Input: part model. Units: mm. Frame: model coordinates. A direction names the side the tool comes from. Round coordinates to 2 decimals unless told otherwise and drop trailing zeros. Loops run counter-clockwise (first coordinate to the right, second up) from the corner with the lowest first, then second, coordinate; pieces in that order, holes last. Notation, with made-up numbers: M -13,29 L 33,29 A15 cw 33,57 Z; hole C 59,-9.5 d3. An arc over 180 degrees is marked long. Return JSON: item names as keys, results as strings. Group by question number.
1) Section D-D (y = -54). Output: boundary loops of the cut face in (x, z).
2) Section B-B (x = 0). Count the separate pieces of the cut face and the enclosed holes in it, plus the area to 3 significant figures.
3) Contact query for flat-ended pins moving along their axis: P1, Ø3, axis at x = 0, z = 0, coming from the +Y side; P2, Ø4, axis at y = -53.5, z = 1.5, coming from the -X side; P3, Ø2, axis at x = 0, y = -56, coming from the +Z side; P4, Ø1.5, axis at x = -3.5, z = 3, coming from the +Y side. Output: stop coordinate, or through.
4) Mould query, pull axis X, two halves, no side actions, for faces 4 (the face through (5.94, -73.819, -1.38)), 5 (the face through (1.38, -75.1, -6.2)), 6 (the face through (-0.05, -41.78, 4.91)). Classes: +X half, -X half, draft (parallel to the pull), parting line (faces both ways), or undercut.
5) Access query for faces 1 (the face through (-5.669, -74.307, 1.785)), 2 (the face through (-0.05, -41.78, -4.8)), 3 (the face through (0, -59, 6.35)). Directions: +Z, -Z, +X, -X, +Y, -Y. A direction counts if a zero-diameter tool reaches every point of the face in a straight line with its end or side. Return the directions, or none.
6) Section A-A (y = -41). Output: boundary loops of the cut face in (x, z).
7) Section C-C (y = -13). Output: boundary loops of the cut face in (x, z).
8) Material intervals for line 1 (X direction, y = -17.75, z = 0); line 2 (X direction, y = -6.5, z = 0); line 3 (Y direction, x = 0.75, z = -6.25), sorted ascending. Write a range as from..to.
from build123d import *

# Parameters (mm, degrees)
F0_R     = 6.35
F0_R_2   = 2.4892
F1_DEPTH = 17.4625
F2_R     = 2.4892
F3_DEPTH = 27.78125
F5_DEPTH = 15.876
F7_DEPTH = 30.1625


with BuildPart() as f1:
    # F0 (on Front) → F1 (new body)
    with BuildSketch(Plane.XZ):
        Circle(F0_R)
        Circle(F0_R_2, mode=Mode.SUBTRACT)
    extrude(amount=F1_DEPTH)

    # F2 (on face) → F3 (join)
    with BuildSketch(Plane.XZ.offset(17.4625)):
        Polygon((4.5827177617, 7.9375), (-4.5827177617, 7.9375), (-9.1654355234, 0), (-4.5827177617, -7.9375), (4.5827177617, -7.9375), (9.1654355234, 0), align=None)
        Circle(F2_R, mode=Mode.SUBTRACT)
    extrude(amount=F3_DEPTH)

    # F4 (on face) → F5 (cut, through all)
    with BuildSketch(Plane.XY.offset(7.9375)):
        with BuildLine():
            ThreePointArc((2.4892, -23.415625), (0, -20.926425), (-2.4892, -23.415625))
            Line((-2.4892, -23.415625), (-2.4892, -39.290625))
            ThreePointArc((-2.4892, -39.290625), (0, -41.779825), (2.4892, -39.290625))
            Line((2.4892, -39.290625), (2.4892, -23.415625))
        make_face()
    extrude(amount=-F5_DEPTH, mode=Mode.SUBTRACT)

    # F6 (on face) → F7 (join)
    with BuildSketch(Plane.XZ.offset(45.24375)):
        Polygon((-3.6661742094, -6.35), (3.6661742094, -6.35), (7.3323484187, 0), (3.6661742094, 6.35), (-3.6661742094, 6.35), (-7.3323484187, 0), align=None)
    extrude(amount=F7_DEPTH)

    # F8 (on Top) → F9 (revolve, cut)
    with BuildSketch(Plane.XY):
        Polygon((-7.3323484187, -75.40625), (-6.35, -75.40625), (-6.35, -74.80935), (-5.9436, -74.80935), (-5.9436, -73.81875), (-7.3323484187, -73.81875), align=None)
        Polygon((6.35, -74.80935), (6.35, -75.40625), (7.3323484187, -75.40625), (7.3323484187, -73.81875), (5.9436, -73.81875), (5.9436, -74.80935), align=None)
        Polygon((7.3323484187, -1.5875), (7.3323484187, 0), (6.35, 0), (6.35, -0.5969), (5.9436, -0.5969), (5.9436, -1.5875), align=None)
        Polygon((-5.9436, -0.5969), (-6.35, -0.5969), (-6.35, 0), (-7.3323484187, 0), (-7.3323484187, -1.5875), (-5.9436, -1.5875), align=None)
    revolve(axis=Axis((0, -37.703125, 0), (0, 1, 0)), mode=Mode.SUBTRACT)


solid = f1.part
Returned:
{
 "1": {"outline": "M -7.33,0 L -3.67,-6.35 L 3.67,-6.35 L 7.33,0 L 3.67,6.35 L -3.67,6.35 Z"},
 "2": {"separate pieces": "3", "enclosed holes": "0", "area": "592 mm^2"},
 "3": {"P1": "stops at y = -45.24", "P2": "stops at x = -7.33", "P3": "stops at z = 6.35", "P4": "stops at y = 0"},
 "4": {"face 4": "draft", "face 5": "parting line", "face 6": "undercut"},
 "5": {"face 1": "none", "face 2": "+Z, -Z", "face 3": "+Z, +X, -X, -Y"},
 "6": {"outline": "M -9.17,0 L -4.58,-7.94 L -1.81,-7.94 L -1.81,-1.71 A2.49 cw -1.81,1.71 L -1.81,7.94 L -4.58,7.94 Z; M 1.81,-7.94 L 4.58,-7.94 L 9.17,0 L 4.58,7.94 L 1.81,7.94 L 1.81,1.71 A2.49 cw 1.81,-1.71 Z"},
 "7": {"outline": "C 0,0 d12.7; hole C 0,0 d4.98"},
 "8": {"line 1": "x = -9.17..-2.49, 2.49..9.17", "line 2": "x = -6.35..-2.49, 2.49..6.35", "line 3": "y = -75.41..-74.81, -73.82..-41.66, -21.04..-1.59, -0.6..0"}
}
